Check sheet for the modelled part. Datum: model origin and axes. Units: mm. Face numbers are marked on the shaded views. A direction names the side the tool comes from. Give positions to 0.01 mm unless a question says otherwise; leave off trailing zeros. Order: outer loops, then holes, each group sorted by start corner. A loop starts at its lowest first (then second) coordinate and runs counter-clockwise, first axis right, second up.
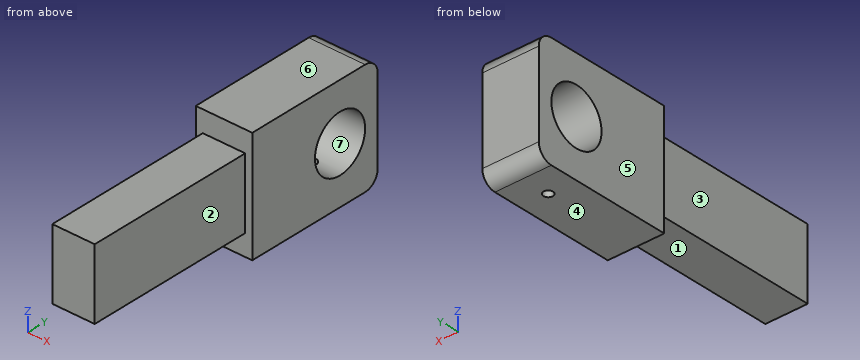
from build123d import *

# Parameters (mm, degrees)
SKETCH2_W               = 19.05
SKETCH2_H               = 31.75
BOSS_EXTRUDE1_DEPTH     = 76.2
SKETCH3_W               = 25.4
SKETCH3_H               = 50.8
BOSS_EXTRUDE2_DEPTH     = 63.5
FILLET1_R               = 6.35
SKETCH4_R               = 12.7
CUT_EXTRUDE1_DEPTH      = 145.244271983
CUT_EXTRUDE2_REACH      = 151.191
CUT_EXTRUDE2_END_RADIUS = 12.7
SKETCH5_R               = 2.15265


with BuildPart() as part:
    # Sketch2 → Boss-Extrude1 (new body)
    with BuildSketch(Plane(origin=(0, 0, 0), x_dir=(1, 0, 0), z_dir=(0, 1, 0))):
        Rectangle(SKETCH2_W, SKETCH2_H)
    extrude(amount=BOSS_EXTRUDE1_DEPTH)

    # Sketch3 → Boss-Extrude2 (add)
    with BuildSketch(Plane(origin=(0, 76.2, 0), x_dir=(1, 0, 0), z_dir=(0, 1, 0))):
        Rectangle(SKETCH3_W, SKETCH3_H)
    extrude(amount=BOSS_EXTRUDE2_DEPTH)

    # Fillet1
    fillet1_edges = [part.edges().sort_by_distance(p)[0] for p in [
        (0, 139.7, -25.4),
        (0, 139.7, 25.4),
    ]]
    fillet(fillet1_edges, radius=FILLET1_R)

    # Sketch4 → Cut-Extrude1 (cut, through all)
    with BuildSketch(Plane(origin=(12.7, 0, 0), x_dir=(0, 0, -1), z_dir=(1, 0, 0))):
        with Locations((0, 120.65)):
            Circle(SKETCH4_R)
    extrude(amount=-CUT_EXTRUDE1_DEPTH, mode=Mode.SUBTRACT)

    # Cut-Extrude2: up to this cylinder (the profile starts outside it)
    cut_extrude2_end = Plane(origin=(0, 120.65, 0), z_dir=(1, 0, 0)) * Cylinder(CUT_EXTRUDE2_END_RADIUS, 328.782, mode=Mode.PRIVATE)
    # Sketch5 → Cut-Extrude2 (cut, up to the surface)
    with BuildSketch(Plane(origin=(0, 0, -25.4), x_dir=(-1, 0, 0), z_dir=(0, 0, -1)), mode=Mode.PRIVATE) as cut_extrude2_sk1:
        with Locations((0, 120.65)):
            Circle(SKETCH5_R)
    cut_extrude2_tool1 = extrude(cut_extrude2_sk1.sketch, amount=-CUT_EXTRUDE2_REACH, mode=Mode.PRIVATE) - cut_extrude2_end
    add(cut_extrude2_tool1.solids().sort_by_distance((0, 120.65, -25.4))[0], mode=Mode.SUBTRACT)


solid = part.part
1) Section check B-B, the plane y = 120.65. Record the cut outline in (x, z), then the cut area to 3 significant figures.
Recorded:
outline: (-12.7, -25.4) - (-2.15, -25.4) - (-2.15, -12.7) - (-12.7, -12.7) - close; (-12.7, 12.7) - (12.7, 12.7) - (12.7, 25.4) - (-12.7, 25.4) - close; (2.15, -25.4) - (12.7, -25.4) - (12.7, -12.7) - (2.15, -12.7) - close
area: 590 mm2
2) Draft check along Z on the marked faces 4, 5, 6 and 7. Enter one of: +Z half, -Z half, draft (parallel to the pull), parting line (faces both ways), or undercut.
Recorded:
face 4: -Z half
face 5: draft
face 6: +Z half
face 7: undercut
3) Section check D-D, the plane z = -6. Record the cut outline in (x, y) (3 decimals).
Recorded:
outline: (-12.7, 76.2) - (-9.525, 76.2) - (-9.525, 0) - (9.525, 0) - (9.525, 76.2) - (12.7, 76.2) - (12.7, 109.457) - (-12.7, 109.457) - close; (-12.7, 131.843) - (12.7, 131.843) - (12.7, 139.7) - (-12.7, 139.7) - close
4) Material ranges on L1, parallel to Y at x = -11, z = 0.5; L2, parallel to Y at x = 0, z = -19.5; L3, parallel to Z at x = 3.75, y = 24.5 (3 decimals), recorded low to high.
Recorded:
L1: y = 76.2 to 107.96, 133.34 to 139.7
L2: y = 76.2 to 118.5, 122.8 to 139.68
L3: z = -15.875 to 15.875
5) Section check C-C, the plane x = 0. Record the cut outline in (y, z) (3 decimals).
Recorded:
outline: (0, -15.875) - (76.2, -15.875) - (76.2, -25.4) - (118.497, -25.4) - (118.497, -12.516) arc R12.7 cw (long way) to (122.803, -12.516) - (122.803, -25.4) - (133.35, -25.4) arc R6.35 ccw to (139.7, -19.05) - (139.7, 19.05) arc R6.35 ccw to (133.35, 25.4) - (76.2, 25.4) - (76.2, 15.875) - (0, 15.875) - close
6) Depth check by flat-ended pin: pin 1 Ø2 at (x, y) = (0.5, 63.5) entering from +Z (3 decimals); pin 2 Ø3.5 at (x, y) = (0, 120.65) entering from -Z; pin 3 Ø1 at (x, z) = (8.5, -19.5) entering from -Y. Enter the tip coordinate at first touch or a pass-through.
Recorded:
pin 1: stops at z = 15.875
pin 2: stops at z = 12.58
pin 3: stops at y = 76.2
7) Section check A-A, the plane z = 0. Record the cut outline in (x, y) (3 decimals), then the cut area to 3 significant figures.
Recorded:
outline: (-12.7, 76.2) - (-9.525, 76.2) - (-9.525, 0) - (9.525, 0) - (9.525, 76.2) - (12.7, 76.2) - (12.7, 107.95) - (-12.7, 107.95) - close; (-12.7, 133.35) - (12.7, 133.35) - (12.7, 139.7) - (-12.7, 139.7) - close
area: 2,420 mm2
8) Set-up check for the marked faces 1, 2 and 3: record each of +Z, -Z, +X, -X, +Y, -Y from which the full face is reachable in a straight line by a thin tool's end or side.
Recorded:
face 1: -Z, +X, -X, -Y
face 2: +Z, -Z, +X, -Y
face 3: +Z, -Z, -X, -Y
